Geometry check sheet. Reference: drawing and pictorial views, mm from the part's lowest x, y, z. A direction names the side the tool comes from. Coordinates: 2 decimals unless noted, no trailing zeros. Order: outer loops, then holes, each group sorted by start corner. A loop starts at its lowest first (then second) coordinate and runs counter-clockwise, first axis right, second up. Notation, with made-up numbers: M -37.5,-31.5 L 20.5,-31.5 A13 ccw 20.5,-8.5 Z; hole C 22.25,15 d7. An arc over 180 degrees is marked long. Return JSON: item names as keys, results as strings.
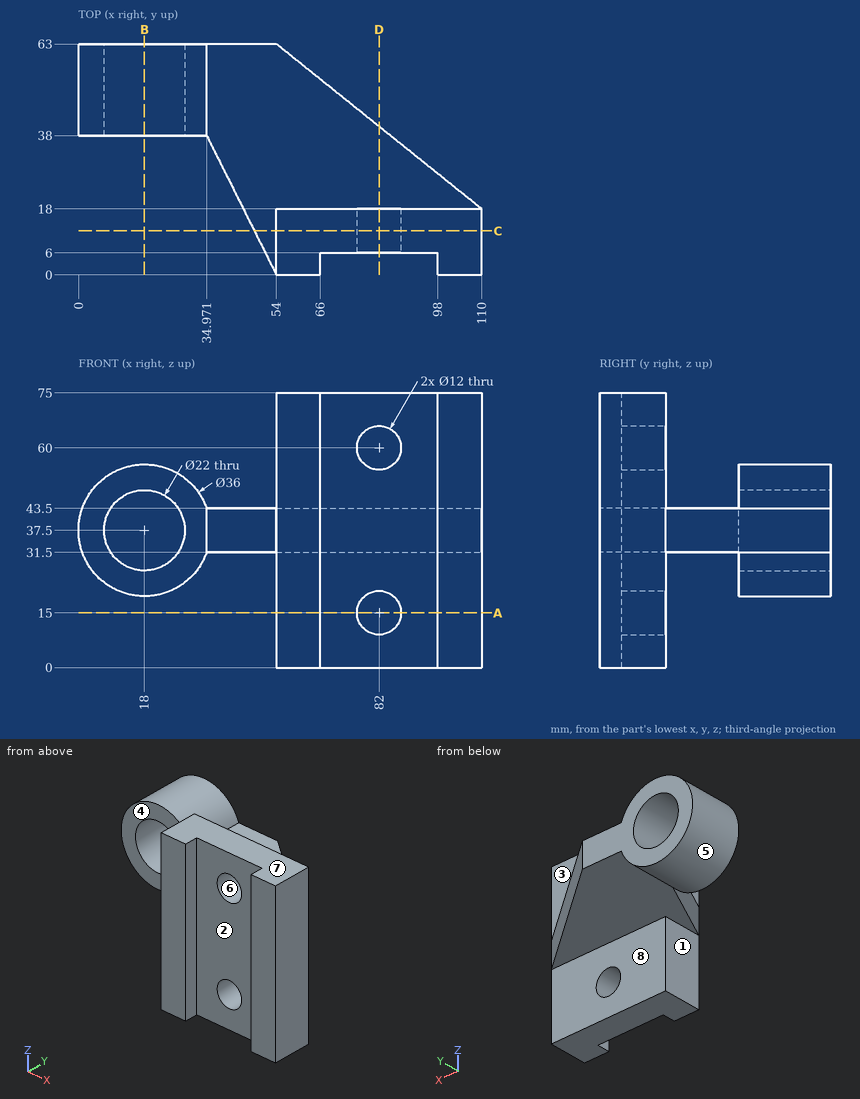
Q1. Cross-section at D-D, the plane x = 82. Record the boundary of the cut face in (y, z).
Values:
{"outline": "M 6,0 L 18,0 L 18,9 L 6,9 Z; M 6,21 L 18,21 L 18,31.5 L 40.5,31.5 L 40.5,43.5 L 18,43.5 L 18,54 L 6,54 Z; M 6,66 L 18,66 L 18,75 L 6,75 Z"}
Q2. Tool access check on the marked faces 1, 2, 3 and 4. Record the directions out of +Z, -Z, +X, -X, +Y, -Y that give a thin tool (end or side, any length) a straight path to the whole face; none if there is none.
Values:
{"face 1": "-Z, -X, +Y, -Y", "face 2": "+Z, -Z, -Y", "face 3": "+Z, +X, -X, +Y", "face 4": "+Z, -Z, -X, -Y"}
Q3. Go/stop test with flat-tipped pins: pin 1 (3 mm diameter, centred on y = 2, z = 40, fed in from -X); pin 2 (9.5 mm diameter, centred on x = 80, z = 50.5, fed in from -Y); pin 3 (20 mm diameter, centred on y = 7.5, z = 62.5, fed in from -X). Record where each tip stops, or that it passes through.
Values:
{"pin 1": "x = 52.25", "pin 2": "y = 6", "pin 3": "x = 54"}
Q4. Cross-section at B-B, the plane x = 18. Record the boundary of the cut face in (y, z), and give its area (3 significant figures).
Values:
{"outline": "M 38,19.5 L 63,19.5 L 63,26.5 L 38,26.5 Z; M 38,48.5 L 63,48.5 L 63,55.5 L 38,55.5 Z", "area": "350 mm^2"}
Q5. Material ranges on line 1 along Z through (x, y) = (82, 12); line 2 along X through (y, z) = (13.75, 15); line 3 along Z through (x, y) = (18, 44), recorded low to high.
Values:
{"line 1": "0 to 9, 21 to 54, 66 to 75", "line 2": "54 to 76, 88 to 110", "line 3": "19.5 to 26.5, 48.5 to 55.5"}
Q6. Draft check along Z on the marked faces 5, 6, 7 and 8. Enter one of: pulls with the +Z half, pulls with the -Z half, needs draft (parallel to the pull), parting line crosses it, or undercut.
Values:
{"face 5": "parting line crosses it", "face 6": "undercut", "face 7": "pulls with the +Z half", "face 8": "needs draft"}
Q7. Cross-section at A-A, the plane z = 15. Record the boundary of the cut face in (x, y), and give its area (3 significant figures).
Values:
{"outline": "M 54,0 L 66,0 L 66,6 L 76,6 L 76,18 L 54,18 Z; M 88,6 L 98,6 L 98,0 L 110,0 L 110,18 L 88,18 Z", "area": "672 mm^2"}
Q8. Cross-section at C-C, the plane y = 12. Record the boundary of the cut face in (x, z).
Values:
{"outline": "M 47.99,31.5 L 54,31.5 L 54,0 L 110,0 L 110,75 L 54,75 L 54,43.5 L 47.99,43.5 Z; hole C 82,15 d12; hole C 82,60 d12"}
